from build123d import *

# Parameters (mm, degrees)
SKETCH1_W               = 211.9
SKETCH1_H               = 38.1
BOSS_EXTRUDE1_DEPTH     = 38.1
SKETCH2_W               = 31.75
SKETCH2_H               = 31.75
CUT_EXTRUDE1_DEPTH      = 1
CUT_EXTRUDE1_DEPTH_BACK = 212.9


with BuildPart() as part:
    # Sketch1 → Boss-Extrude1 (new body)
    with BuildSketch(Plane.XY):
        with Locations((105.95, 19.05)):
            Rectangle(SKETCH1_W, SKETCH1_H)
    extrude(amount=-BOSS_EXTRUDE1_DEPTH)

    # Sketch2 → Cut-Extrude1 (cut, two sides)
    with BuildSketch(Plane(origin=(211.9, 0, 0), x_dir=(0, 0, -1), z_dir=(1, 0, 0))) as cut_extrude1_sk:
        with Locations((19.05, 19.05)):
            Rectangle(SKETCH2_W, SKETCH2_H)
    extrude(amount=CUT_EXTRUDE1_DEPTH, mode=Mode.SUBTRACT)
    extrude(cut_extrude1_sk.sketch, amount=-CUT_EXTRUDE1_DEPTH_BACK, mode=Mode.SUBTRACT)


solid = part.part
CAD build for the part. Positions are in the model's coordinates, mm. A direction names the side the tool comes from. Round coordinates to 2 decimals unless told otherwise and drop trailing zeros. Order: outer loops, then holes, each group sorted by start corner. A loop starts at its lowest first (then second) coordinate and runs counter-clockwise, first axis right, second up. Notation, with made-up numbers: (44.5, -39.75) -> (62.5, -39.75) arc R5 ccw to (62.5, -34.75) -> close; hole circle Ø4 at (-5.5, 38.25). An arc over 180 degrees is marked (long way). Write each question's results on one line, items separated by ' | '.
1. Pull direction Y, two halves, no side cores. Call faces 1 (the face through (211.9, 36, -19)), 2 (the face through (107, 19, -3.175)), 3 (the face through (104, 0, -19)), 4 (the face through (107, 34.925, -19)): pulls with the +Y half, pulls with the -Y half, needs draft (parallel to the pull), parting line crosses it, or undercut.
Findings below:
face 1: needs draft | face 2: undercut | face 3: pulls with the -Y half | face 4: undercut
2. Cut at A-A (y = 32.5). Give the cut face in (x, z) (3 decimals), plus the area to 3 significant figures.
Findings below:
outline: (0, -38.1) -> (211.9, -38.1) -> (211.9, -34.925) -> (0, -34.925) -> close; (0, -3.175) -> (211.9, -3.175) -> (211.9, 0) -> (0, 0) -> close | area: 1,350 mm²
3. Cut at B-B (z = -20.5). Give the cut face in (x, y) (3 decimals).
Findings below:
outline: (0, 0) -> (211.9, 0) -> (211.9, 3.175) -> (0, 3.175) -> close; (0, 34.925) -> (211.9, 34.925) -> (211.9, 38.1) -> (0, 38.1) -> close
4. Cut at C-C (x = 45). Give the cut face in (y, z) (3 decimals), plus the area to 3 significant figures.
Findings below:
outline: (0, -38.1) -> (38.1, -38.1) -> (38.1, 0) -> (0, 0) -> close; hole (3.175, -34.925) -> (34.925, -34.925) -> (34.925, -3.175) -> (3.175, -3.175) -> close | area: 444 mm²
5. Wall check: line 1 along Y through (x, z) = (157, -27) (3 decimals); line 2 along Z through (x, y) = (60.5, 19.5) (3 decimals). Give the ranges that are in metal, low to high. Write a range as [from, to].
Findings below:
line 1: y = [0, 3.175], [34.925, 38.1] | line 2: z = [-38.1, -34.925], [-3.175, 0]
6. 3-axis set-ups, long thin cutter, end or side, ignore diameter. For faces 5 (the face through (0, 36, -19)), 6 (the face through (107, 3.175, -19)): which of +Z, -Z, +X, -X, +Y, -Y reach the whole face in a straight line?
Findings below:
face 5: +Z, -Z, -X, +Y, -Y | face 6: +X, -X
